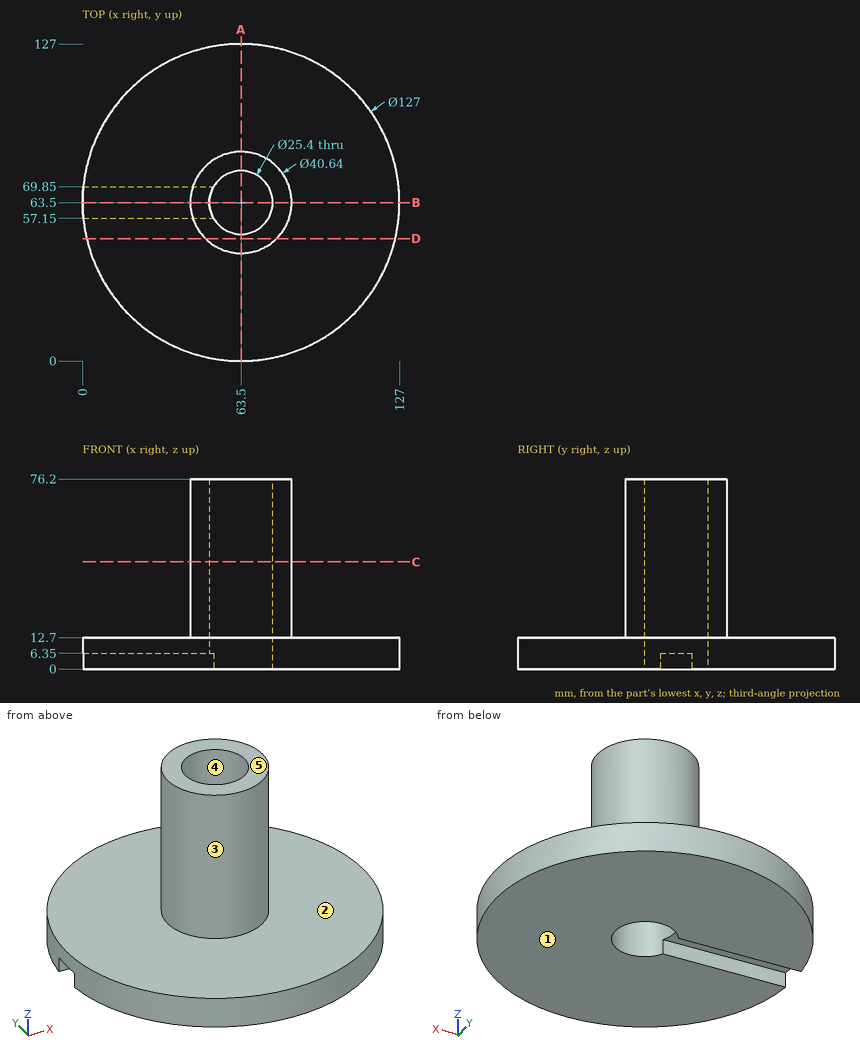
Geometry: see drawing. Coordinates: mm, zero at the bounding-box minimum. A direction names the side the tool comes from. Coordinates: 2 decimals unless noted, no trailing zeros. Write each loop counter-clockwise with the first axis right and the second up, starting at its lowest first coordinate (ties: lowest second). Pieces come first, ordered by that corner, then holes. Notation, with made-up numbers: M -22.5,-17 L 3.5,-17 A17 ccw 3.5,2 Z; hole C -20,54.5 d1. An arc over 180 degrees is marked long. Use CSV: the item, a comma, the result in double quotes. Start each with the question number.
1. Mould query, pull axis Y, two halves, no side actions, for the marked faces 3, 4 and 5. Classes: pulls with the +Y half, pulls with the -Y half, needs draft (parallel to the pull), parting line crosses it, or undercut.
2. Cut plane D-D on y = 49. Return the cut outline in (x, z), plus the area to 3 significant figures.
3. Ray query, probe 1 along X at (y, z) = (63, 55); probe 2 along Z at (x, y) = (92.5, 35.5). Return the intervals inside material, ascending.
4. Cut plane B-B on y = 63.5. Return the cut outline in (x, z).
5. Cut plane A-A on x = 63.5. Return the cut outline in (y, z), plus the area to 3 significant figures.
6. First-contact query: P1, Ø12, axis at x = 112, y = 30.5, coming from the -Z side; P2, Ø1.9, axis at x = 36, z = 3, coming from the -Y side; P3, Ø5, axis at x = 24.5, z = 3.5, coming from the +Y side; P4, Ø8, axis at x = 74, z = 53.5, coming from the +Y side. Flat tips, straight axial feed; report the tip coordinate or a pass-through.
7. Reachability of the marked faces 1 and 2 from +Z, -Z, +X, -X, +Y, -Y: full face, straight path, thin tool, end or side. Return the list, or none.
8. Cut plane C-C on z = 43. Return the cut outline in (x, y).
Entries:
1,face 3,"parting line crosses it"
1,face 4,"undercut"
1,face 5,"needs draft"
2,outline,"M 1.68,0 L 125.32,0 L 125.32,12.7 L 77.74,12.7 L 77.74,76.2 L 49.26,76.2 L 49.26,12.7 L 1.68,12.7 Z"
2,area,"3,380 mm²"
3,probe 1,"43.19 to 50.81, 76.19 to 83.81"
3,probe 2,"0 to 12.7"
4,outline,"M 0,6.35 L 50.8,6.35 L 50.8,76.2 L 43.18,76.2 L 43.18,12.7 L 0,12.7 Z; M 76.2,0 L 127,0 L 127,12.7 L 83.82,12.7 L 83.82,76.2 L 76.2,76.2 Z"
5,outline,"M 0,0 L 50.8,0 L 50.8,76.2 L 43.18,76.2 L 43.18,12.7 L 0,12.7 Z; M 76.2,0 L 127,0 L 127,12.7 L 83.82,12.7 L 83.82,76.2 L 76.2,76.2 Z"
5,area,"2,260 mm²"
6,P1,"z = 0"
6,P2,"y = 5.82"
6,P3,"y = 115.46"
6,P4,"y = 82.75"
7,face 1,"-Z, +X, -X, +Y, -Y"
7,face 2,"+Z"
8,outline,"C 63.5,63.5 d40.64; hole C 63.5,63.5 d25.4"
